Design review of the part built by this model. Coordinates are the model's own, in mm. A direction names the side the tool comes from. Coordinates: 2 decimals unless noted, no trailing zeros. Loops run counter-clockwise (first coordinate to the right, second up) from the corner with the lowest first, then second, coordinate; pieces in that order, holes last.
Q1. Add section C-C on y = 22.25. Give the boundary of the cut face in (x, z), and give its area (3 significant figures).
Q2. Machinability: for faces 5 (the face through (1, 0, -7)), 6 (the face through (1.46, 12.17, -16.49)), 7 (the face through (1.5, 4, 5)), 8 (the face through (0, 12, -10.965)), 9 (the face through (0.5, 12, -26)), which of the approach directions +Z, -Z, +X, -X, +Y, -Y give a long, thin tool a straight path to every point of the face, cutting with its end or side? Answer none if there is none.
Q3. Draft analysis for pull direction Y (two halves, no side actions). For faces 1 (the face through (4.5, 12, -25)), 2 (the face through (1, 24, -7)), 3 (the face through (0, 19, 5)), 4 (the face through (0, 5, 5)), state which applies: released by +Y, released by -Y, zero draft, split by the parting line, or undercut.
Q4. For P1, Ø3.5, axis at x = 0.5, y = 12, coming from the -Z side; P2, Ø10, axis at y = 17, z = -4, coming from the +X side; P3, Ø0.9, axis at x = 0.5, y = 14, coming from the +Z side, all flat-tipped, find the tip position at first contact; note any pin that passes through.
Q5. Wall thickness on probe 1 along Y at (x, z) = (-0.75, -3); probe 2 along Z at (x, y) = (-0.25, 5.25); probe 3 along X at (y, z) = (22, -26): over which ranges is each line inside the solid? List them lowest first.
Q6. Add section A-A on z = 10. Give the boundary of the cut face in (x, y).
Q7. Add section B-B on y = 10. Give the boundary of the cut face in (x, z), and give its area (3 significant figures).
```python
from build123d import *

# Parameters (mm, degrees)
BOSS_EXTRUDE1_DEPTH = 24
CUT_EXTRUDE1_DEPTH  = 24
FILLET5_R           = 1
FILLET6_R           = 5.5
FILLET8_R           = 2
SKETCH3_W           = 32.464758902
SKETCH3_H           = 14
CUT_EXTRUDE2_DEPTH  = 10
FILLET9_R           = 5


with BuildPart() as part:
    # Sketch1 → Boss-Extrude1 (new body)
    with BuildSketch(Plane(origin=(0, 0, 0), x_dir=(1, 0, 0), z_dir=(0, 1, 0))):
        Polygon((1.5, 36.5), (5.9, 39.627739059), (5.9, 15.124617794), (1.5, 11.996878735), (1.5, -26.5), (-1.5, -26.5), (-1.5, 36.5), align=None)
    extrude(amount=BOSS_EXTRUDE1_DEPTH)

    # Sketch2 → Cut-Extrude1 (cut)
    with BuildSketch(Plane(origin=(0, 24, 0), x_dir=(1, 0, 0), z_dir=(0, 1, 0))):
        with BuildLine():
            Line((-1.5, 14.383985508), (4.5, 18.649084224))
            Line((4.5, 18.649084224), (4.5, 31.313323891))
            ThreePointArc((4.5, 31.313323891), (2.5, 33.313323891), (0.5, 31.313323891))
            Line((0.5, 31.313323891), (0.5, 20.713323891))
            Line((0.5, 20.713323891), (-1.5, 19.291624318))
            Line((-1.5, 19.291624318), (-1.5, 14.383985508))
        make_face()
    extrude(amount=-CUT_EXTRUDE1_DEPTH, mode=Mode.SUBTRACT)

    # Fillet5
    fillet5_edges = [part.edges().sort_by_distance(p)[0] for p in [
        (-1.5, 12, -14.383985508),
        (0.5, 12, -20.713323891),
        (4.5, 12, -18.649084224),
    ]]
    fillet(fillet5_edges, radius=FILLET5_R)

    # Fillet6
    # the kernel refuses this fillet: 5.5 mm, written as the material it takes off along each edge
    with BuildSketch(Plane(origin=(-1.5, -12.247448714, -36.5), x_dir=(0, 0, 1), z_dir=(0, 1, 0))) as fillet6_piece_1:
        with BuildLine():
            CenterArc((4.898979486, 5.5), FILLET6_R, 207.035691789, 62.964308211)
            Line((0, 3), (-0.09797959, 2.95))
            ThreePointArc((-0.09797959, 2.95), (-0.11, 1.5), (-0.11, 0))
            Line((-0.11, 0), (0, -0.11))
            Line((0, -0.11), (4.898979486, -0.11))
            Line((4.898979486, -0.11), (4.898979486, 0))
        make_face()
    extrude(amount=48.494897428, mode=Mode.SUBTRACT)

    # Fillet8
    fillet8_edges = [part.edges().sort_by_distance(p)[0] for p in [
        (5.9, 12, -15.124617794),
        (1.5, 12, -11.996878735),
    ]]
    fillet(fillet8_edges, radius=FILLET8_R)

    # Sketch3 → Cut-Extrude2 (cut)
    with BuildSketch(Plane(origin=(1.5, 0, 0), x_dir=(0, 0, -1), z_dir=(1, 0, 0))):
        with Locations((-5.267620549, 12)):
            Rectangle(SKETCH3_W, SKETCH3_H)
    extrude(amount=-CUT_EXTRUDE2_DEPTH, mode=Mode.SUBTRACT)

    # Fillet9
    # the kernel refuses this fillet: 5 mm, written as the material it takes off along each edge
    with BuildSketch(Plane(origin=(1.5, -11.456439237, 26.5), x_dir=(0, 0, -1), z_dir=(0, 1, 0))) as fillet9_piece_1:
        with BuildLine():
            CenterArc((4.582575695, 5), FILLET9_R, 203.578178478, 66.421821522)
            Line((0, 3), (-0.091651514, 2.96))
            ThreePointArc((-0.091651514, 2.96), (-0.1, 1.5), (-0.1, 0))
            Line((-0.1, 0), (0, -0.1))
            Line((0, -0.1), (4.582575695, -0.1))
            Line((4.582575695, -0.1), (4.582575695, 0))
        make_face()
    extrude(amount=46.912878475, mode=Mode.SUBTRACT)


solid = part.part
```
Entries:
1. outline: (-1.5, -31.6) arc R5.5 ccw to (1.5, -36.5) - (5.9, -39.63) - (5.9, -16.16) arc R2 ccw to (5.06, -14.53) - (2.34, -12.59) arc R2 cw to (1.5, -10.96) - (1.5, 21.92) arc R5 ccw to (-1.5, 26.5) - (-1.5, -13.87) arc R1 ccw to (-1.08, -14.68) - (4.08, -18.35) arc R1 cw to (4.5, -19.17) - (4.5, -31.31) arc R2 cw to (0.5, -31.31) - (0.5, -21.23) arc R1 ccw to (0.08, -20.41) - (-1.5, -19.29) - close
1. area: 216 mm2
2. face 5: +Z, -Z, +X, -X, -Y
2. face 6: -X, +Y, -Y
2. face 7: +Z, +X, +Y, -Y
2. face 8: +X, -X
2. face 9: +Y, -Y
3. face 1: zero draft
3. face 2: released by +Y
3. face 3: undercut
3. face 4: undercut
4. P1: stops at z = -37.03
4. P2: stops at x = 1.5
4. P3: stops at z = 25.44
5. probe 1: y = 0 to 5, 19 to 24
5. probe 2: z = -35.09 to -20.18, -15.27 to -10.96, 21.5 to 25.72
5. probe 3: x = -1.5 to 0.5, 4.5 to 5.9
6. outline: (-1.5, 0) - (1.5, 0) - (1.5, 5) - (-1.5, 5) - close; (-1.5, 19) - (1.5, 19) - (1.5, 24) - (-1.5, 24) - close
7. outline: (-1.5, -31.6) arc R5.5 ccw to (1.5, -36.5) - (5.9, -39.63) - (5.9, -16.16) arc R2 ccw to (5.06, -14.53) - (2.34, -12.59) arc R2 cw to (1.5, -10.96) - (-1.5, -10.96) - (-1.5, -13.87) arc R1 ccw to (-1.08, -14.68) - (4.08, -18.35) arc R1 cw to (4.5, -19.17) - (4.5, -31.31) arc R2 cw to (0.5, -31.31) - (0.5, -21.23) arc R1 ccw to (0.08, -20.41) - (-1.5, -19.29) - close; (-1.5, 21.5) - (1.5, 21.5) - (1.5, 21.92) arc R5 ccw to (-1.5, 26.5) - close
7. area: 119 mm2
